Verification items for the finished model (mm, model axes). A direction names the side the tool comes from. Coordinates: 2 decimals unless noted, no trailing zeros. Write each loop counter-clockwise with the first axis right and the second up, starting at its lowest first coordinate (ties: lowest second). Pieces come first, ordered by that corner, then holes. Notation, with made-up numbers: M 10,76.5 L 43,76.5 A29 cw 43,112.5 Z; hole C -7,34.5 d1. An arc over 180 degrees is marked long. One line per item, written item: value.
```python
from build123d import *

# Parameters (mm, degrees)
F1_DEPTH = 62
F2_R     = 11.7474696308
F3_DEPTH = 62
F5_DEPTH = 62
F6_R     = 10.330572445
F7_DEPTH = 62


with BuildPart() as f1:
    # F0 (on Right) → F1 (new body)
    with BuildSketch(Plane.YZ):
        Polygon((72.0315793902, 5.5999404844), (-47.9684206098, 5.5999404844), (-47.9684206098, -14.4000595156), (72.0315793902, -14.4000595156), (72.0315793902, -4.4000595156), align=None)
        Polygon((-47.9684206098, -14.4000595156), (-47.9684206098, 5.5999404844), (-108.6771392604, 47.9136673329), (-116.9353204182, 29.6982221294), align=None)
    extrude(amount=F1_DEPTH)

    # F2 (on Right) → F3 (join)
    with BuildSketch(Plane.YZ):
        with Locations((-111.1419275403, 36.2391285598)):
            Circle(F2_R)
    extrude(amount=F3_DEPTH)

    # F4 (on face) → F5 (cut)
    with BuildSketch(Plane.XY.offset(5.5999404844)):
        with BuildLine():
            ThreePointArc((21.8113110218, 51.0349926195), (31.9204424494, 41.3457998855), (41.7515892409, 51.316935569))
            ThreePointArc((41.7515892409, 51.316935569), (31.6384713179, 61.2880712526), (21.8113110218, 51.0349926195))
        make_face()
        with BuildLine():
            Line((42.6100902259, 51.316935569), (41.7515892409, 51.316935569))
            ThreePointArc((41.7515892409, 51.316935569), (31.9204424494, 41.3457998855), (21.8113110218, 51.0349926195))
            Line((21.8113110218, 51.0349926195), (23.3906661796, -4.8034051943))
            ThreePointArc((23.3906661796, -4.8034051943), (32.9119310697, 1.8000949809), (42.6100902259, -4.540757379))
            Line((42.6100902259, -4.540757379), (42.6100902259, 51.316935569))
        make_face()
        with BuildLine():
            ThreePointArc((43.4248242139, -8.5701132193), (43.2191003354, -6.5146631494), (42.6100902259, -4.540757379))
            Line((42.6100902259, -4.540757379), (42.6100902259, -8.5701132193))
            Line((42.6100902259, -8.5701132193), (23.4972052276, -8.5701132193))
            Line((23.4972052276, -8.5701132193), (23.3906661796, -4.8034051943))
            ThreePointArc((23.3906661796, -4.8034051943), (31.1372951092, -18.7627033893), (43.4248242139, -8.5701132193))
        make_face()
        with BuildLine():
            Line((42.6100902259, -8.5701132193), (42.6100902259, -4.540757379))
            ThreePointArc((42.6100902259, -4.540757379), (32.9119310697, 1.8000949809), (23.3906661796, -4.8034051943))
            Line((23.3906661796, -4.8034051943), (23.4972052276, -8.5701132193))
            Line((23.4972052276, -8.5701132193), (42.6100902259, -8.5701132193))
        make_face()
    extrude(amount=-F5_DEPTH, mode=Mode.SUBTRACT)

    # F6 (on face) → F7 (cut)
    with BuildSketch(Plane(origin=(0, -13.0569639472, -18.7332010139), x_dir=(1, 0, 0), z_dir=(0, 0.5718071196, 0.8203880899))):
        with Locations((31, -93.1249111891)):
            Circle(F6_R)
    extrude(amount=-F7_DEPTH, mode=Mode.SUBTRACT)


solid = f1.part
```
Item 1: Cross-section at B-B, the plane y = 35.5. Enter the section's corners in (x, z), and give its area (3 significant figures).
The answers:
outline: M 0,-14.4 L 22.25,-14.4 L 22.25,5.6 L 0,5.6 Z; M 42.61,-14.4 L 62,-14.4 L 62,5.6 L 42.61,5.6 Z
area: 833 mm²
Item 2: Scan lines: line 1 (Z direction, x = 53.5, y = 48); line 2 (X direction, y = 30, z = 1); line 3 (X direction, y = -85.5, z = 30.5). Record each from-to range of solid material in increasing order.
The answers:
line 1: z = -14.4 to 5.6
line 2: x = 0 to 22.41, 42.61 to 62
line 3: x = 0 to 22.28, 39.72 to 62
Item 3: Access from +Z, -Z, +X, -X, +Y, -Y to the whole of each face (thin tool, end or side, straight path). Record for faces 5 (the face through (31, 72.032, -5)), 6 (the face through (31.86, 61.29, -4.26)), 7 (the face through (17, 13, 5.6)).
The answers:
face 5: +Z, -Z, +X, -X, +Y
face 6: +Z, -Z
face 7: +Z, +X, -X, +Y
Item 4: Cross-section at C-C, the plane x = 9.5. Enter the section's corners in (y, z).
The answers:
outline: M -109.08,24.67 L -47.97,-14.4 L 72.03,-14.4 L 72.03,5.6 L -47.97,5.6 L -101.45,42.88 A11.75 ccw -108.27,47.63 L -108.68,47.91 L -108.76,47.74 A11.75 ccw long Z
Item 5: Draft check along X on faces 1 (the face through (30.566, -104.376, 45.842)), 2 (the face through (62, -26, 3)), 3 (the face through (0, -26, 3)), 4 (the face through (42.61, 23, -4)). Enter one of: released by +X, released by -X, zero draft, split by the parting line, or undercut.
The answers:
face 1: zero draft
face 2: released by +X
face 3: released by -X
face 4: undercut
Item 6: Go/stop test with flat-tipped pins: P1, Ø12, axis at x = 29.5, y = -43.5, coming from the +Z side; P2, Ø4, axis at x = 31, z = 23, coming from the +Y side; P3, Ø8, axis at x = 9, z = -1, coming from the -Y side; P4, Ø1, axis at x = 16, z = 36, coming from the -Y side. Record where each tip stops, or that it passes through.
The answers:
P1: stops at z = 6.67
P2: stops at y = -70.06
P3: stops at y = -75.18
P4: stops at y = -122.89
Item 7: Cross-section at D-D, the plane z = -9.5. Enter the section's corners in (x, y) (3 decimals), and give its area (3 significant figures).
The answers:
outline: M 0,-55.632 L 62,-55.632 L 62,72.032 L 0,72.032 Z; hole M 21.811,51.035 L 23.391,-4.803 A10.371 ccw long 42.61,-4.541 L 42.61,51.317 L 41.752,51.317 A9.972 ccw long Z
area: 6,390 mm²
Item 8: Cross-section at A-A, the plane x = 31.5. Enter the section's corners in (y, z).
The answers:
outline: M -109.08,24.67 L -108.95,24.59 L -97.92,40.42 L -101.45,42.88 A11.75 ccw -108.27,47.63 L -108.68,47.91 L -108.76,47.74 A11.75 ccw long Z; M -91.55,13.47 L -47.97,-14.4 L -18.82,-14.4 L -18.82,5.6 L -47.97,5.6 L -80.99,28.62 Z; M 61.29,-14.4 L 72.03,-14.4 L 72.03,5.6 L 61.29,5.6 Z
